from build123d import *

# Parameters (mm, degrees)
SKETCH29_R              = 1.1
SKETCH29_R_2            = 1.075
BOSS_EXTRUDE19_DEPTH    = 2.5
SKETCH31_R              = 1.1
CUT_EXTRUDE2_DEPTH      = 2.5
SKETCH15_W              = 3.25
SKETCH15_H              = 15
SKETCH15_W_2            = 2.7
BOSS_EXTRUDE11_DEPTH    = 15
FILLET10_R              = 7.5
CUT_EXTRUDE1_DEPTH      = 12
CUT_EXTRUDE1_DEPTH_BACK = 17
SKETCH16_R              = 2.7
BOSS_EXTRUDE12_START    = 2.1
SKETCH17_R              = 5.5
SKETCH17_R_2            = 2.7
BOSS_EXTRUDE12_DEPTH    = 2.1
BOSS_EXTRUDE17_DEPTH    = 3
FILLET11_R              = 3
FILLET12_R              = 10


with BuildPart() as part:
    # Sketch29 → Boss-Extrude19 (new body)
    with BuildSketch(Plane(origin=(0, 0, 0), x_dir=(1, 0, 0), z_dir=(0, 1, 0))):
        with BuildLine():
            Line((-15, -70), (15, -70))
            Line((15, -70), (15, -30.089902911))
            ThreePointArc((15, -30.089902911), (18.35, -27), (15, -23.910097089))
            Line((15, -23.910097089), (15, 50))
            Line((15, 50), (-15, 50))
            Line((-15, 50), (-15, -23.910097089))
            ThreePointArc((-15, -23.910097089), (-18.35, -27), (-15, -30.089902911))
            Line((-15, -30.089902911), (-15, -70))
        make_face()
        with Locations(Location((-15.25, -27, 0), (0, 0, 270))):
            Circle(SKETCH29_R, mode=Mode.SUBTRACT)
        with Locations(Location((-13, 13, 0), (0, 0, 270))):
            Circle(SKETCH29_R_2, mode=Mode.SUBTRACT)
        with Locations(Location((13, 13, 0), (0, 0, 270))):
            Circle(SKETCH29_R_2, mode=Mode.SUBTRACT)
        with Locations(Location((13, -13, 0), (0, 0, 270))):
            Circle(SKETCH29_R_2, mode=Mode.SUBTRACT)
        with Locations(Location((-13, -13, 0), (0, 0, 270))):
            Circle(SKETCH29_R_2, mode=Mode.SUBTRACT)
        with Locations(Location((15.25, -27, 0), (0, 0, 270))):
            Circle(SKETCH29_R, mode=Mode.SUBTRACT)
    extrude(amount=BOSS_EXTRUDE19_DEPTH)

    # Sketch31 → Cut-Extrude2 (cut)
    with BuildSketch(Plane(origin=(0, 2.5, 0), x_dir=(1, 0, 0), z_dir=(0, 1, 0))):
        with Locations(Location((-10, -45, 0), (0, 0, 270))):
            Circle(SKETCH31_R)
        with Locations(Location((10, -45, 0), (0, 0, 270))):
            Circle(SKETCH31_R)
        with Locations(Location((-10, 45, 0), (0, 0, 270))):
            Circle(SKETCH31_R)
        with Locations(Location((10, 45, 0), (0, 0, 270))):
            Circle(SKETCH31_R)
    extrude(amount=-CUT_EXTRUDE2_DEPTH, mode=Mode.SUBTRACT)

    # Sketch15 → Boss-Extrude11 (add)
    with BuildSketch(Plane(origin=(0, 2.5, 0), x_dir=(1, 0, 0), z_dir=(0, 1, 0))):
        with Locations((0, 38)):
            Rectangle(SKETCH15_W, SKETCH15_H)
        with Locations((-6.125, 38)):
            Rectangle(SKETCH15_W_2, SKETCH15_H)
        with Locations((6.125, 38)):
            Rectangle(SKETCH15_W_2, SKETCH15_H)
    extrude(amount=BOSS_EXTRUDE11_DEPTH)

    # Fillet10
    fillet10_edges = [part.edges().sort_by_distance(p)[0] for p in [
        (6.125, 17.5, -30.5),
        (6.125, 17.5, -45.5),
        (0, 17.5, -30.5),
        (0, 17.5, -45.5),
        (-6.125, 17.5, -30.5),
        (-6.125, 17.5, -45.5),
    ]]
    fillet(fillet10_edges, radius=FILLET10_R - 0.0001)  # a hair under: the kernel refuses the full size

    # Sketch16 → Cut-Extrude1 (cut, two sides: drawn at the far end of the back side and taken through both)
    with BuildSketch(Plane.ZY.offset(7.475).offset(-CUT_EXTRUDE1_DEPTH_BACK)):
        with Locations(Location((-38, 10, 0), (0, 0, 180))):
            Circle(SKETCH16_R)
    extrude(amount=CUT_EXTRUDE1_DEPTH + CUT_EXTRUDE1_DEPTH_BACK, mode=Mode.SUBTRACT)

    # Sketch17 → Boss-Extrude12 (add)
    with BuildSketch(Plane.ZY.offset(7.475).offset(BOSS_EXTRUDE12_START)):
        with Locations(Location((-38, 10, 0), (0, 0, 180))):
            Circle(SKETCH17_R)
        with Locations(Location((-38, 10, 0), (0, 0, 180))):
            Circle(SKETCH17_R_2, mode=Mode.SUBTRACT)
    extrude(amount=-BOSS_EXTRUDE12_DEPTH)

    # Sketch23 → Boss-Extrude17 (add)
    with BuildSketch(Plane(origin=(7.475, 0, 0), x_dir=(0, 0, -1), z_dir=(1, 0, 0))):
        Polygon((38, 16.350852961), (32.5, 13.175426481), (32.5, 6.824573519), (38, 3.649147039), (43.5, 6.824573519), (43.5, 13.175426481), align=None)
        Polygon((38, 14.618802154), (34, 12.309401077), (34, 7.690598923), (38, 5.381197846), (42, 7.690598923), (42, 12.309401077), align=None, mode=Mode.SUBTRACT)
    extrude(amount=BOSS_EXTRUDE17_DEPTH)

    # Fillet11
    fillet11_edges = [part.edges().sort_by_distance(p)[0] for p in [
        (15, 1.25, 23.910097089),
        (15, 1.25, 30.089902911),
        (-15, 1.25, 30.089902911),
        (-15, 1.25, 23.910097089),
    ]]
    fillet(fillet11_edges, radius=FILLET11_R)

    # Fillet12
    fillet12_edges = [part.edges().sort_by_distance(p)[0] for p in [
        (15, 1.25, 70),
        (-15, 1.25, 70),
    ]]
    fillet(fillet12_edges, radius=FILLET12_R)


solid = part.part
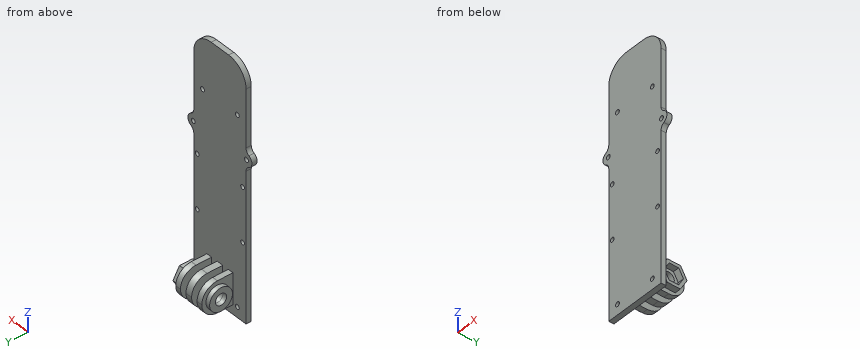
Geometry: final body of the model. Coordinates: model frame, mm. Give positions to 0.01 mm unless a question says otherwise; leave off trailing zeros. Order: outer loops, then holes, each group sorted by start corner. A loop starts at its lowest first (then second) coordinate and runs counter-clockwise, first axis right, second up. Notation, with made-up numbers: (36, -33) -> (56, -33) arc R20 ccw to (56, -13) -> close; hole circle Ø5 at (34, -11.75). An arc over 180 degrees is marked (long way). Write each question's results on one line, items separated by ' | '.
1) Cut plane A-A (z = 13). Output: boundary loops of the cut face in (x, y) (3 decimals).
Geometry says:
outline: (-15, 0) -> (-14.075, 0) -> (-14.075, 2.5) -> (-15, 2.5) -> close; (-11.925, 0) -> (11.925, 0) -> (11.925, 2.5) -> (-11.925, 2.5) -> close; (14.075, 0) -> (15, 0) -> (15, 2.5) -> (14.075, 2.5) -> close
2) Line query: line 1 along X through (y, z) = (12.75, -33.5) (3 decimals); line 2 along X through (y, z) = (1.05, 13) (3 decimals); line 3 along Y through (x, z) = (6, -38). Output: solid intervals per line, ascending.
Geometry says:
line 1: x = -9.575 to -4.775, -1.625 to 1.625, 4.775 to 10.475 | line 2: x = -15 to -14.075, -11.925 to 11.925, 14.075 to 15 | line 3: y = 0 to 7.3, 12.7 to 17.5
3) First-contact query: pin 1 Ø1.5 at (x, z) = (3, 43.5) entering from +Y; pin 2 Ø2.5 at (x, z) = (15.25, 27) entering from -Y; pin 3 Ø7.5 at (y, z) = (8.5, -38.5) entering from +X (3 decimals); pin 4 Ø3 at (x, y) = (10, 6.5) entering from +Z. Flat tips, straight axial feed; report the tip coordinate or a pass-through.
Geometry says:
pin 1: stops at y = 2.5 | pin 2: stops at y = 0 | pin 3: stops at x = 10.475 | pin 4: stops at z = -32.5
4) Cut plane B-B (x = -13). Output: boundary loops of the cut face in (y, z) (3 decimals), and give its area (3 significant figures).
Geometry says:
outline: (0, -50) -> (2.5, -50) -> (2.5, -14.075) -> (0, -14.075) -> close; (0, -11.925) -> (2.5, -11.925) -> (2.5, 11.925) -> (0, 11.925) -> close; (0, 14.075) -> (2.5, 14.075) -> (2.5, 66) -> (0, 66) -> close | area: 279 mm²
